```python
from build123d import *

# Parameters (mm, degrees)
F1_DEPTH = 24.638
F2_R     = 13.015145
F2_R_2   = 12.398002
F3_DEPTH = 35.052


with BuildPart() as f1:
    # F0 (on Right) → F1 (new body)
    with BuildSketch(Plane.YZ):
        with BuildLine():
            Line((-109.188519, -41.18206), (-109.269887, -15.63245))
            ThreePointArc((-109.269887, -15.63245), (-127.226123, -59.277199), (-83.63878, -41.18206))
            Line((-83.63878, -41.18206), (-109.188519, -41.18206))
        make_face()
        with BuildLine():
            ThreePointArc((-83.63878, -41.18206), (-91.150916, -23.086921), (-109.269887, -15.63245))
            Line((-109.269887, -15.63245), (-109.188519, -41.18206))
            Line((-109.188519, -41.18206), (-83.63878, -41.18206))
        make_face()
        with BuildLine():
            Line((-78.279719, 44.706121), (-109.462045, 44.706121))
            Line((-109.462045, 44.706121), (-109.269887, -15.63245))
            ThreePointArc((-109.269887, -15.63245), (-91.150916, -23.086921), (-83.63878, -41.18206))
            Line((-83.63878, -41.18206), (39.820287, -41.18206))
            ThreePointArc((39.820287, -41.18206), (47.289896, -23.148827), (65.323129, -15.679217))
            Line((65.323129, -15.679217), (65.323129, 44.706121))
            Line((65.323129, 44.706121), (-7.162113, 14.617906))
            Line((-7.162113, 14.617906), (-45.182679, 14.617906))
            Line((-45.182679, 14.617906), (-78.279719, 44.706121))
        make_face()
        with BuildLine():
            Line((65.323129, -41.18206), (39.820287, -41.18206))
            ThreePointArc((39.820287, -41.18206), (65.323129, -66.684902), (90.825972, -41.18206))
            ThreePointArc((90.825972, -41.18206), (83.356362, -23.148827), (65.323129, -15.679217))
            Line((65.323129, -15.679217), (65.323129, -41.18206))
        make_face()
        with BuildLine():
            ThreePointArc((65.323129, -15.679217), (47.289896, -23.148827), (39.820287, -41.18206))
            Line((39.820287, -41.18206), (65.323129, -41.18206))
            Line((65.323129, -41.18206), (65.323129, -15.679217))
        make_face()
    extrude(amount=F1_DEPTH)

    # F2 (on face) → F3 (cut)
    with BuildSketch(Plane.YZ.offset(24.638)):
        with Locations((-109.188519, -41.18206)):
            Circle(F2_R)
        with Locations((65.323129, -41.18206)):
            Circle(F2_R_2)
    extrude(amount=-F3_DEPTH, mode=Mode.SUBTRACT)


solid = f1.part
```
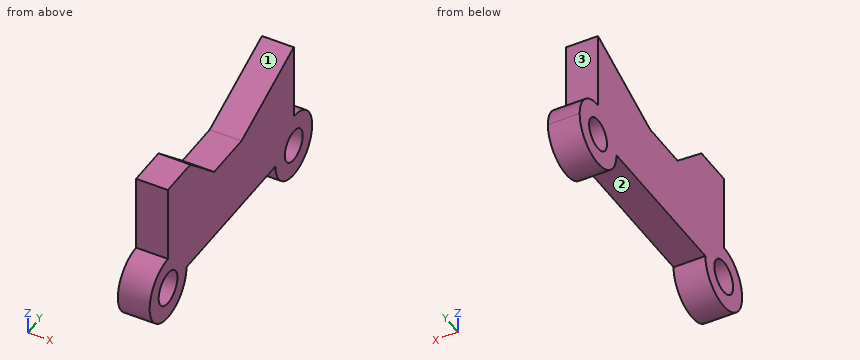
Design review of the part built by this model. Coordinates are the model's own, in mm. Face numbers are marked on the shaded views. A direction names the side the tool comes from. Give positions to 0.01 mm unless a question says otherwise; leave off trailing zeros. Order: outer loops, then holes, each group sorted by start corner. A loop starts at its lowest first (then second) coordinate and runs counter-clockwise, first axis right, second up. Notation, with made-up numbers: (16, 52) -> (21, 52) arc R17 cw to (21, 81) -> close; hole circle Ø6 at (-6, -16.75). An arc over 180 degrees is marked (long way). Write item = value, one per line. Start each with the question number.
(1) To check wall thickness, follow line 1 along Y through (x, z) = (17, -34.5); line 2 along Z through (x, y) = (6.5, -23.5); line 3 along Y through (x, z) = (7.5, 22.5). State the ranges of each line that lie inside material, in increasing order.
(2) For pin 1 (4 mm diameter, centred on y = -43, z = -5.5, fed in from -X); pin 2 (2 mm diameter, centred on x = 10, y = 22, fed in from +Z); pin 3 (2 mm diameter, centred on x = 14.5, z = 26.5, fed in from -Y); pin 4 (8 mm diameter, centred on x = 12.5, z = 0.5, fed in from +Y), all flat-tipped, find the tip position at first contact; note any pin that passes through.
(3) We need section A-A on z = 18. Write out the cut boundary in (x, y), plus the area to 3 significant figures.
(4) For the marked faces 1, 2 and 3, list the 3-axis set-ups (+Z, -Z, +X, -X, +Y, -Y) from which the entire face can be reached by the end or side of a thin tool; tool diameter is ignored.
(5) We need section C-C on z = -50. Write out the cut boundary in (x, y).
(6) We need section B-B on x = 11. Write out the cut boundary in (y, z), plus the area to 3 significant figures.
(7) We need section D-D on y = -25. Write out the cut boundary in (x, z), plus the area to 3 significant figures.
Numbers:
q1.line_1 = -133.85 to -120.36, -98.02 to 54.88, 75.77 to 89.94
q1.line_2 = -41.18 to 14.62
q1.line_3 = -109.39 to -53.85, 11.83 to 65.32
q2.pin_1 = 0
q2.pin_2 = 27.14
q2.pin_3 = -109.41
q2.pin_4 = 65.32
q3.outline = (0, -109.38) -> (24.64, -109.38) -> (24.64, -48.9) -> (0, -48.9) -> close; (0, 0.99) -> (24.64, 0.99) -> (24.64, 65.32) -> (0, 65.32) -> close
q3.area = 3,080 mm^2
q4.face_1 = +Z, +X, -X
q4.face_2 = -Z, +X, -X
q4.face_3 = +Z, +X, -X, +Y
q5.outline = (0, -133.17) -> (24.64, -133.17) -> (24.64, -118.76) -> (0, -118.76) -> close; (0, -99.62) -> (24.64, -99.62) -> (24.64, -85.21) -> (0, -85.21) -> close; (0, 41.39) -> (24.64, 41.39) -> (24.64, 56.61) -> (0, 56.61) -> close; (0, 74.04) -> (24.64, 74.04) -> (24.64, 89.25) -> (0, 89.25) -> close
q6.outline = (-109.46, 44.71) -> (-109.27, -15.63) arc R25.55 ccw (long way) to (-83.64, -41.18) -> (39.82, -41.18) arc R25.5 ccw to (90.83, -41.18) arc R25.5 ccw to (65.32, -15.68) -> (65.32, 44.71) -> (-7.16, 14.62) -> (-45.18, 14.62) -> (-78.28, 44.71) -> close; hole circle Ø26.03 at (-109.19, -41.18); hole circle Ø24.8 at (65.32, -41.18)
q6.area = 14,300 mm^2
q7.outline = (0, -41.18) -> (24.64, -41.18) -> (24.64, 14.62) -> (0, 14.62) -> close
q7.area = 1,370 mm^2
